from build123d import *

# Parameters (mm, degrees)
F0_W     = 3
F0_H     = 6
F2_R     = 3
F3_DEPTH = 15


# Not quite as in the source:
# - a feature names something its author has since deleted; it is built from what else it names


with BuildPart() as f1:
    # F0 (on Front) → F1 (revolve)
    with BuildSketch(Plane.XZ):
        with BuildLine():
            Line((-5.5, 35), (-14.375, 35))
            Line((-14.375, 35), (-14.375, -35))
            Line((-14.375, -35), (0, -35))
            Line((0, -35), (0, -30.075))
            ThreePointArc((0, -30.075), (-7.1241008205, -27.1241008205), (-10.075, -20))
            Line((-10.075, -20), (-12.375, -20))
            Line((-12.375, -20), (-12.375, -0.2))
            Line((-12.375, -0.2), (-10.075, -0.2))
            Line((-10.075, -0.2), (-10.075, 20))
            ThreePointArc((-10.075, 20), (-7.9590553774, 26.1773022024), (-2.5, 29.7598988212))
            Line((-2.5, 29.7598988212), (-2.5, 35))
            Line((-2.5, 35), (-5.5, 35))
        make_face()
        with Locations((-4, 38)):
            Rectangle(F0_W, F0_H)
    revolve(axis=Axis((0, 0, 0), (0, 0, -1)))

    # F2 (on Front) → F3 (cut, symmetric)
    with BuildSketch(Plane.XZ):
        with Locations((0, -10.2)):
            Circle(F2_R)
    extrude(amount=F3_DEPTH, both=True, mode=Mode.SUBTRACT)


solid = f1.part
For this review, take the finished solid that the model builds, in its own axes (mm). A direction names the side the tool comes from. Round coordinates to 2 decimals unless told otherwise and drop trailing zeros. Loops run counter-clockwise (first coordinate to the right, second up) from the corner with the lowest first, then second, coordinate; pieces in that order, holes last. Notation, with made-up numbers: (38, -40) - (86, -40) arc R26 cw to (86, -23) - close; hole circle Ø2 at (-23, 54.25). An arc over 180 degrees is marked (long way). One line per question, with ' | ' between items.
Q1. Take a section at C-C (z = -10.2). Give the boundary of the cut face in (x, y) (3 decimals).
Taken from the geometry:
outline: (-3, -14.058) - (-3, -12.006) arc R12.375 cw to (-3, 12.006) - (-3, 14.058) arc R14.375 ccw to start; (3, -14.058) arc R14.375 ccw to (3, 14.058) - (3, 12.006) arc R12.375 cw to (3, -12.006) - close
Q2. Take a section at D-D (x = -7). Give the boundary of the cut face in (y, z).
Taken from the geometry:
outline: (-12.56, -35) - (12.56, -35) - (12.56, 35) - (-12.56, 35) - close; hole (-10.2, -20) - (-7.25, -20) arc R7.25 ccw to (7.25, -20) - (10.2, -20) - (10.2, -0.2) - (7.25, -0.2) - (7.25, 20) arc R7.25 ccw to (-7.25, 20) - (-7.25, -0.2) - (-10.2, -0.2) - close
Q3. For line 1 along Z through (x, y) = (-10, -5); line 2 along Z through (x, y) = (0, -13.65); line 3 along Y through (x, z) = (0, 36.25), list the stretches that pass through material, from the lowest coordinate up. Write a range as [from, to].
Taken from the geometry:
line 1: z = [-35, -20], [-0.2, 35] | line 2: z = [-35, -13.2], [-7.2, 35] | line 3: y = [-5.5, -2.5], [2.5, 5.5]
Q4. Take a section at A-A (x = 0). State how many separate pieces and enclosed holes the cut face has, and give its area (3 significant figures).
Taken from the geometry:
separate pieces: 3 | enclosed holes: 0 | area: 783 mm²
Q5. For pin 1 (8 mm diameter, centred on x = 4.5, z = 32.5, fed in from +Y); pin 2 (3 mm diameter, centred on y = -4, z = -2.5, fed in from +X); pin 3 (1.5 mm diameter, centred on x = 7.5, z = -2.5, fed in from -Y), all flat-tipped, find the tip position at first contact; note any pin that passes through.
Taken from the geometry:
pin 1: stops at y = 14.37 | pin 2: stops at x = 14.16 | pin 3: stops at y = -12.69
Q6. The part is to be moulded in two halves that separate along Z. For faces 4 (the flat face through (5, -9, -0.2)), 5 (the cylindrical face through (0.54, -2.44, 35.46)), 6 (the flat face through (3, 0, 41)), say which applies: released by +Z, released by -Z, zero draft, split by the parting line, or undercut.
Taken from the geometry:
face 4: undercut | face 5: zero draft | face 6: released by +Z
Q7. Take a section at B-B (y = 0). Give the boundary of the cut face in (x, z) (3 decimals).
Taken from the geometry:
outline: (-14.375, -35) - (14.375, -35) - (14.375, 35) - (5.5, 35) - (5.5, 41) - (2.5, 41) - (2.5, 29.76) arc R10.075 cw to (10.075, 20) - (10.075, -0.2) - (12.375, -0.2) - (12.375, -20) - (10.075, -20) arc R10.075 cw to (-10.075, -20) - (-12.375, -20) - (-12.375, -0.2) - (-10.075, -0.2) - (-10.075, 20) arc R10.075 cw to (-2.5, 29.76) - (-2.5, 41) - (-5.5, 41) - (-5.5, 35) - (-14.375, 35) - close
Q8. Tool access review of faces 1 (the cylindrical face through (-9.307, -3.859, 10.041)), 2 (the cylindrical face through (2.77, 13.18, -11.35)), 3 (the cylindrical face through (1.19, -5.37, 38.04)): name each direction out of +Z, -Z, +X, -X, +Y, -Y from which nothing blocks a thin tool from reaching the whole face with its end or side.
Taken from the geometry:
face 1: none | face 2: +Y, -Y | face 3: +Z
